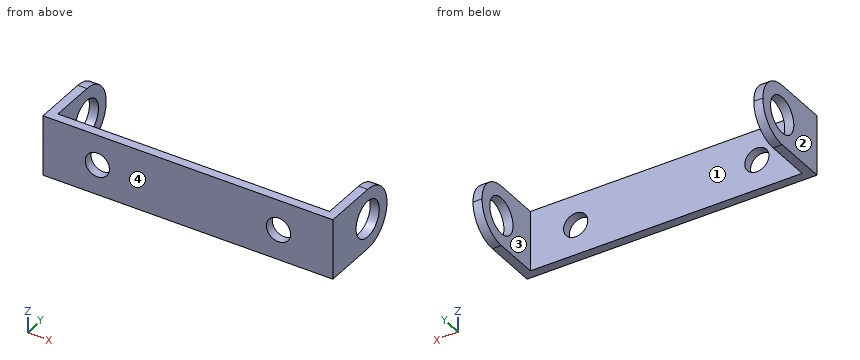
```python
from build123d import *

# Parameters (mm, degrees)
BOSS_EXTRUDE1_DEPTH = 10
CUT_EXTRUDE1_REACH  = 51.528
SKETCH3_R           = 2
CUT_EXTRUDE2_DEPTH  = 10


with BuildPart() as part:
    # Sketch1 → Boss-Extrude1 (new body)
    with BuildSketch(Plane.XY):
        Polygon((-22.5, 7), (-22.5, -5.5), (22.5, -5.5), (22.5, 7), (24, 7), (24, -7), (-24, -7), (-24, 7), align=None)
    extrude(amount=BOSS_EXTRUDE1_DEPTH)

    # Cut-Extrude1: up to this face of the body (flat: up to its plane)
    cut_extrude1_end = Plane(part.part.faces().sort_by_distance((-24, 0, 5))[0])
    # Sketch2 → Cut-Extrude1 (cut, up to the picked face)
    with BuildSketch(Plane(origin=(24, 0, 0), x_dir=(0, 0, -1), z_dir=(1, 0, 0)), mode=Mode.PRIVATE) as cut_extrude1_sk1:
        with BuildLine():
            ThreePointArc((-10, 2), (-8.535533906, 5.535533906), (-5, 7))
            Line((-5, 7), (-10, 7))
            Line((-10, 7), (-10, 2))
        make_face()
    cut_extrude1_tool1 = split(extrude(cut_extrude1_sk1.sketch, amount=-CUT_EXTRUDE1_REACH, mode=Mode.PRIVATE), bisect_by=cut_extrude1_end, keep=Keep.BOTH, mode=Mode.PRIVATE)
    # Sketch2 → Cut-Extrude1 (cut, up to the picked face)
    with BuildSketch(Plane(origin=(24, 0, 0), x_dir=(0, 0, -1), z_dir=(1, 0, 0)), mode=Mode.PRIVATE) as cut_extrude1_sk2:
        with BuildLine():
            ThreePointArc((-5, 7), (-1.464466094, 5.535533906), (0, 2))
            Line((0, 2), (0, 7))
            Line((0, 7), (-5, 7))
        make_face()
    cut_extrude1_tool2 = split(extrude(cut_extrude1_sk2.sketch, amount=-CUT_EXTRUDE1_REACH, mode=Mode.PRIVATE), bisect_by=cut_extrude1_end, keep=Keep.BOTH, mode=Mode.PRIVATE)
    # Sketch2 → Cut-Extrude1 (cut, up to the picked face)
    with BuildSketch(Plane(origin=(24, 0, 0), x_dir=(0, 0, -1), z_dir=(1, 0, 0)), mode=Mode.PRIVATE) as cut_extrude1_sk3:
        with BuildLine():
            ThreePointArc((-8, 2), (-5, -1), (-2, 2))
            Line((-2, 2), (-8, 2))
        make_face()
    cut_extrude1_tool3 = split(extrude(cut_extrude1_sk3.sketch, amount=-CUT_EXTRUDE1_REACH, mode=Mode.PRIVATE), bisect_by=cut_extrude1_end, keep=Keep.BOTH, mode=Mode.PRIVATE)
    # Sketch2 → Cut-Extrude1 (cut, up to the picked face)
    with BuildSketch(Plane(origin=(24, 0, 0), x_dir=(0, 0, -1), z_dir=(1, 0, 0)), mode=Mode.PRIVATE) as cut_extrude1_sk4:
        with BuildLine():
            Line((-8, 2), (-2, 2))
            ThreePointArc((-2, 2), (-5, 5), (-8, 2))
        make_face()
    cut_extrude1_tool4 = split(extrude(cut_extrude1_sk4.sketch, amount=-CUT_EXTRUDE1_REACH, mode=Mode.PRIVATE), bisect_by=cut_extrude1_end, keep=Keep.BOTH, mode=Mode.PRIVATE)
    # Sketch2 → Cut-Extrude1 (cut, up to the picked face)
    with BuildSketch(Plane(origin=(24, 0, 0), x_dir=(0, 0, -1), z_dir=(1, 0, 0)), mode=Mode.PRIVATE) as cut_extrude1_sk5:
        with BuildLine():
            ThreePointArc((-8, 2), (-5, -1), (-2, 2))
            Line((-2, 2), (-8, 2))
        make_face()
    cut_extrude1_tool5 = split(extrude(cut_extrude1_sk5.sketch, amount=-CUT_EXTRUDE1_REACH, mode=Mode.PRIVATE), bisect_by=cut_extrude1_end, keep=Keep.BOTH, mode=Mode.PRIVATE)
    # Sketch2 → Cut-Extrude1 (cut, up to the picked face)
    with BuildSketch(Plane(origin=(24, 0, 0), x_dir=(0, 0, -1), z_dir=(1, 0, 0)), mode=Mode.PRIVATE) as cut_extrude1_sk6:
        with BuildLine():
            Line((-8, 2), (-2, 2))
            ThreePointArc((-2, 2), (-5, 5), (-8, 2))
        make_face()
    cut_extrude1_tool6 = split(extrude(cut_extrude1_sk6.sketch, amount=-CUT_EXTRUDE1_REACH, mode=Mode.PRIVATE), bisect_by=cut_extrude1_end, keep=Keep.BOTH, mode=Mode.PRIVATE)
    add(cut_extrude1_tool1.solids().sort_by(Axis((24, 5.88316, 8.88316), (-1, 0, 0)))[0], mode=Mode.SUBTRACT)
    add(cut_extrude1_tool2.solids().sort_by(Axis((24, 5.88316, 1.11684), (-1, 0, 0)))[0], mode=Mode.SUBTRACT)
    add(cut_extrude1_tool3.solids().sort_by(Axis((24, 0.72676, 5), (-1, 0, 0)))[0], mode=Mode.SUBTRACT)
    add(cut_extrude1_tool4.solids().sort_by(Axis((24, 3.27324, 5), (-1, 0, 0)))[0], mode=Mode.SUBTRACT)
    add(cut_extrude1_tool5.solids().sort_by(Axis((24, 0.72676, 5), (-1, 0, 0)))[0], mode=Mode.SUBTRACT)
    add(cut_extrude1_tool6.solids().sort_by(Axis((24, 3.27324, 5), (-1, 0, 0)))[0], mode=Mode.SUBTRACT)

    # Sketch3 → Cut-Extrude2 (cut)
    with BuildSketch(Plane(origin=(0, -5.5, 0), x_dir=(1, 0, 0), z_dir=(0, 1, 0))):
        with Locations(Location((15, -5, 0), (0, 0, 270))):
            Circle(SKETCH3_R)
        with Locations(Location((-15, -5, 0), (0, 0, 270))):
            Circle(SKETCH3_R)
    extrude(amount=-CUT_EXTRUDE2_DEPTH, mode=Mode.SUBTRACT)


solid = part.part
```
Work out the finished part from the listing and answer in its coordinate system (mm). Face numbers are marked on the shaded views. Coordinates: 2 decimals unless noted, no trailing zeros. Write each loop counter-clockwise with the first axis right and the second up, starting at its lowest first coordinate (ties: lowest second). Pieces come first, ordered by that corner, then holes.
Q1. A cutting plane is placed at A-A, the plane y = -4. Give the vertices of the cut face in (x, z), then the cut area to 3 significant figures.
Q2. A cutting plane is placed at B-B, the plane x = -15. Give the vertices of the cut face in (y, z).
Q3. Find the intervals of material crossed by line 1 (X direction, y = -6.45, z = 5); line 2 (Y direction, x = -23.6, z = 5); line 3 (X direction, y = -4.75, z = 4.75), in increasing order.
Q4. Determine the mould class of the marked faces 1, 2, 3 and 4 for opening direction X: released by +X, released by -X, zero draft, split by the parting line, or undercut.
Q5. A cutting plane is placed at D-D, the plane x = 10. Give the vertices of the cut face in (y, z), then the cut area to 3 significant figures.
Q6. A cutting plane is placed at C-C, the plane y = 3.75. Give the vertices of the cut face in (x, z), then the cut area to 3 significant figures.
Findings below:
1. outline: (-24, 0) - (-22.5, 0) - (-22.5, 10) - (-24, 10) - close; (22.5, 0) - (24, 0) - (24, 10) - (22.5, 10) - close
1. area: 30.0 mm2
2. outline: (-7, 0) - (-5.5, 0) - (-5.5, 3) - (-7, 3) - close; (-7, 7) - (-5.5, 7) - (-5.5, 10) - (-7, 10) - close
3. line 1: x = -24 to -17, -13 to 13, 17 to 24
3. line 2: y = -7 to -1, 5 to 7
3. line 3: x = -24 to -22.5, 22.5 to 24
4. face 1: undercut
4. face 2: released by -X
4. face 3: undercut
4. face 4: zero draft
5. outline: (-7, 0) - (-5.5, 0) - (-5.5, 10) - (-7, 10) - close
5. area: 15.0 mm2
6. outline: (-24, 0.32) - (-22.5, 0.32) - (-22.5, 2.56) - (-24, 2.56) - close; (-24, 7.44) - (-22.5, 7.44) - (-22.5, 9.68) - (-24, 9.68) - close; (22.5, 0.32) - (24, 0.32) - (24, 2.56) - (22.5, 2.56) - close; (22.5, 7.44) - (24, 7.44) - (24, 9.68) - (22.5, 9.68) - close
6. area: 13.5 mm2
